Geometry check sheet. Reference: drawing and pictorial views, mm from the part's lowest x, y, z. A direction names the side the tool comes from. Coordinates: 2 decimals unless noted, no trailing zeros. Write each loop counter-clockwise with the first axis right and the second up, starting at its lowest first coordinate (ties: lowest second). Pieces come first, ordered by that corner, then holes. Notation, with made-up numbers: (-7.5, -11.75) -> (12.5, -11.75) arc R14 ccw to (12.5, -3.75) -> close; hole circle Ø7 at (2, 13). An arc over 180 degrees is marked (long way). Use a Markdown table: item, result.
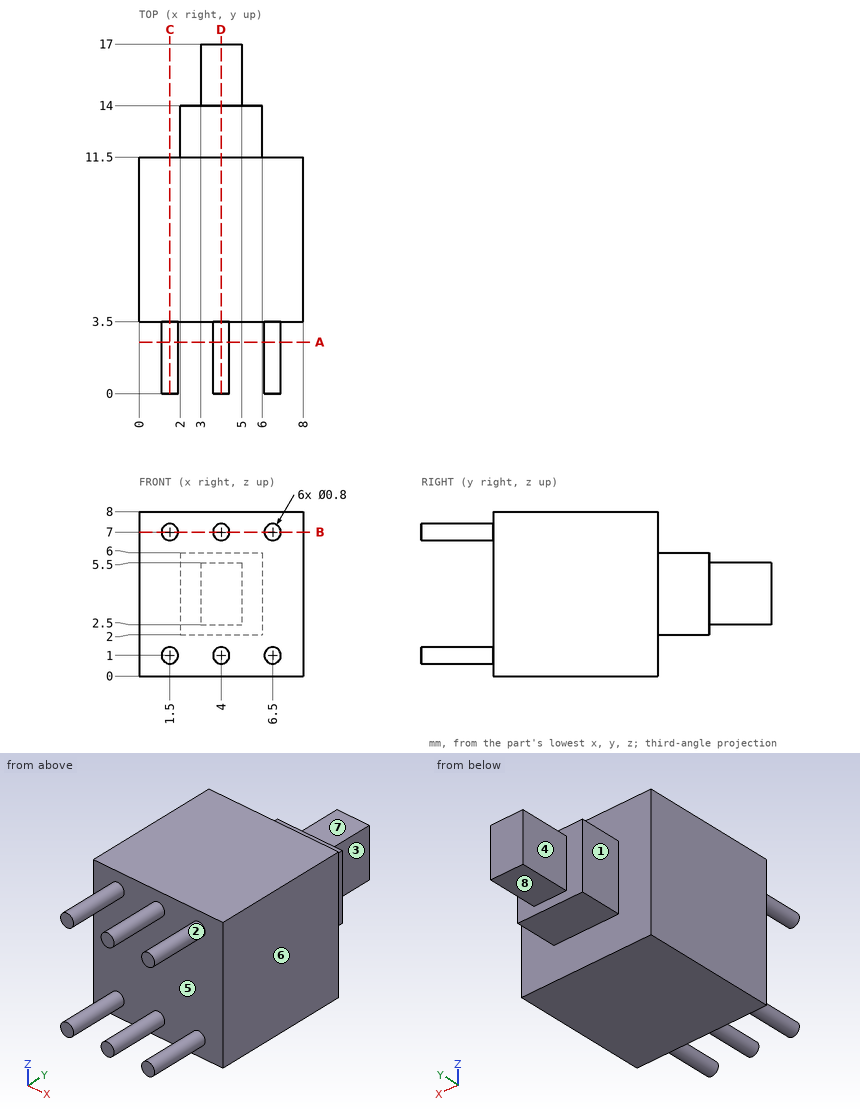
Item 1: Thickness scan on L1, parallel to Y at x = 2.25, z = 2.25; L2, parallel to Z at x = 6.75, y = 2; L3, parallel to Y at x = 7.25, z = 1. Record the ranges inside material, lowest first. Write a range as [from, to].
Answer block:
| item | result |
|---|---|
| L1 | y = [3.5, 14] |
| L2 | z = [0.69, 1.31], [6.69, 7.31] |
| L3 | y = [3.5, 11.5] |
Item 2: Mould release check, pull along X, two halves, no side actions. Record for the marked faces 1, 2 and 3: +X half, -X half, draft (parallel to the pull), parting line (faces both ways), or undercut.
Answer block:
| item | result |
|---|---|
| face 1 | -X half |
| face 2 | undercut |
| face 3 | +X half |
Item 3: Section check A-A on y = 2.5. Record the boundary of the cut face in (x, z), then the cut area to 3 significant figures.
Answer block:
| item | result |
|---|---|
| outline | circle Ø0.8 at (1.5, 1); circle Ø0.8 at (1.5, 7); circle Ø0.8 at (4, 1); circle Ø0.8 at (4, 7); circle Ø0.8 at (6.5, 1); circle Ø0.8 at (6.5, 7) |
| area | 3.02 mm^2 |
Item 4: Section check C-C on x = 1.5. Record the boundary of the cut face in (y, z), then the cut area to 3 significant figures.
Answer block:
| item | result |
|---|---|
| outline | (0, 0.6) -> (3.5, 0.6) -> (3.5, 0) -> (11.5, 0) -> (11.5, 8) -> (3.5, 8) -> (3.5, 7.4) -> (0, 7.4) -> (0, 6.6) -> (3.5, 6.6) -> (3.5, 1.4) -> (0, 1.4) -> close |
| area | 69.6 mm^2 |
Item 5: Depth check by flat-ended pin: P1, Ø4, axis at x = 2, y = 2, coming from the +Z side; P2, Ø0.8, axis at x = 4.5, y = 13.5, coming from the -Z side; P3, Ø1.2, axis at y = 12.5, z = 5, coming from the -X side; P4, Ø2.5, axis at y = 15.5, z = 3.5, coming from the -X side. Enter the tip coordinate at first touch or a pass-through.
Answer block:
| item | result |
|---|---|
| P1 | stops at z = 8 |
| P2 | stops at z = 2 |
| P3 | stops at x = 2 |
| P4 | stops at x = 3 |
Item 6: Section check B-B on z = 7. Record the boundary of the cut face in (x, y), then the cut area to 3 significant figures.
Answer block:
| item | result |
|---|---|
| outline | (0, 3.5) -> (1.1, 3.5) -> (1.1, 0) -> (1.9, 0) -> (1.9, 3.5) -> (3.6, 3.5) -> (3.6, 0) -> (4.4, 0) -> (4.4, 3.5) -> (6.1, 3.5) -> (6.1, 0) -> (6.9, 0) -> (6.9, 3.5) -> (8, 3.5) -> (8, 11.5) -> (0, 11.5) -> close |
| area | 72.4 mm^2 |
Item 7: Section check D-D on x = 4. Record the boundary of the cut face in (y, z).
Answer block:
| item | result |
|---|---|
| outline | (0, 0.6) -> (3.5, 0.6) -> (3.5, 0) -> (11.5, 0) -> (11.5, 2) -> (14, 2) -> (14, 2.5) -> (17, 2.5) -> (17, 5.5) -> (14, 5.5) -> (14, 6) -> (11.5, 6) -> (11.5, 8) -> (3.5, 8) -> (3.5, 7.4) -> (0, 7.4) -> (0, 6.6) -> (3.5, 6.6) -> (3.5, 1.4) -> (0, 1.4) -> close |
Item 8: Tool access check on the marked faces 4, 5, 6, 7 and 8. Record the directions out of +Z, -Z, +X, -X, +Y, -Y that give a thin tool (end or side, any length) a straight path to the whole face; none if there is none.
Answer block:
| item | result |
|---|---|
| face 4 | +Z, -Z, -X, +Y |
| face 5 | -Y |
| face 6 | +Z, -Z, +X, +Y, -Y |
| face 7 | +Z, +X, -X, +Y |
| face 8 | -Z, +X, -X, +Y |
